CAD build for the part. Positions are in the model's coordinates, mm. Face numbers are marked on the shaded views. A direction names the side the tool comes from. Coordinates: 2 decimals unless noted, no trailing zeros. Order: outer loops, then holes, each group sorted by start corner. A loop starts at its lowest first (then second) coordinate and runs counter-clockwise, first axis right, second up. Notation, with made-up numbers: (-16.5, 84.5) - (42.5, 84.5) arc R19 ccw to (42.5, 108.5) - close; hole circle Ø6 at (24.5, 47). An arc over 180 degrees is marked (long way). Write each question's results on one line, items separated by ' | '. Start each with the question number.
Q1. Band-saw the part on B-B, the plane x = 4.5. Write the cut outline in (y, z).
Q2. Band-saw the part on A-A, the plane y = -22. Write the cut outline in (x, z).
Q3. Pin check, flat tips, straight feed: P1, Ø1.1, axis at x = 9.5, z = 59.5, coming from the -Y side; P2, Ø0.5, axis at x = 5, z = 59, coming from the +Y side; P3, Ø1, axis at y = 32.5, z = 52, coming from the -X side. Stop position of each tip, or through.
Q4. Band-saw the part on C-C, the plane z = 22.5. Write the cut outline in (x, y).
Q5. Which spindle directions (+Z, -Z, +X, -X, +Y, -Y) get a long thin tool onto all of the face, cutting with end or side? Do the marked faces 1, 2 and 3. Say none if no direction does.
Q6. Wall check: probe 1 along Z at (x, y) = (6.25, -47.5); probe 2 along X at (y, z) = (8, 29.5); probe 3 along X at (y, z) = (-48, 61.5). Give the ranges that are in metal, low to high.
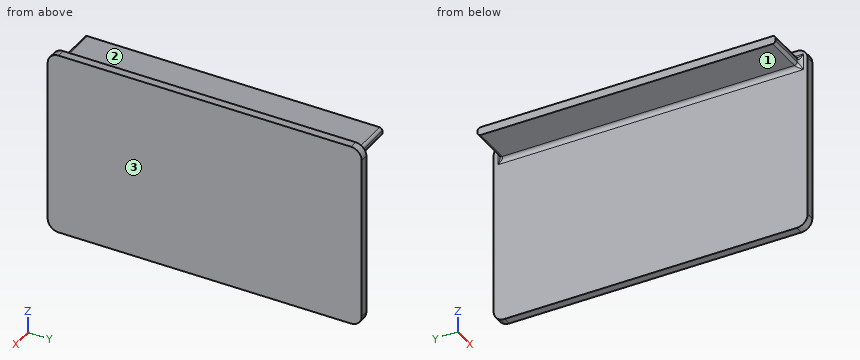
Autodesk Fusion 360 part; units mm, degrees
sketch "Boceto1" plane through (0, 0, 0) normal (1, 0, 0) x (0, 1, 0)
  line L0 (-54.5, 54) -> (54.5, 54)
  line L1 (54.5, 54) -> (54.5, 0)
  line L2 (54.5, 0) -> (-54.5, 0)
  line L3 (-54.5, 0) -> (-54.5, 54)
  dimension "d4" = 54
  dimension "d5" = 109
extrude "Extruir1" add sketch "Boceto1" along normal blind 14 makes body 1
sketch "Boceto2" plane through (0, 0, 0) normal (-1, 0, 0) x (0, -1, 0)
  line L0 (-54.5, 0) -> (54.5, 0)
  line L1 (54.5, 0) -> (54.5, 54)
  line L2 (54.5, 54) -> (-54.5, 54)
  line L3 (-54.5, 54) -> (-54.5, 0)
  line L4 (-58, -3.5) -> (-58, 64.2)
  line L5 (-58, 64.2) -> (-51.5, 64.2)
  line L6 (-51.5, 64.2) -> (-51.5, 61.2)
  line L7 (-51.5, 61.2) -> (-55, 61.2)
  line L8 (-55, 61.2) -> (-55, 57.5)
  line L9 (-55, 57.5) -> (-51.5, 57.5)
  line L10 (-51.5, 57.5) -> (-51.5, 54.5)
  line L11 (-51.5, 54.5) -> (-55, 54.5)
  line L12 (-55, 54.5) -> (-55, -0.5)
  line L13 (-55, -0.5) -> (0, -0.5)
  line L14 (-58, -3.5) -> (0, -3.5)
  line L15 (0, 2.5) -> (0, 20)
  line L16 (58, -3.5) -> (0, -3.5)
  line L17 (55, -0.5) -> (0, -0.5)
  line L18 (55, 54.5) -> (55, -0.5)
  line L19 (58, -3.5) -> (58, 64.2)
  line L20 (51.5, 54.5) -> (55, 54.5)
  line L21 (51.5, 57.5) -> (51.5, 54.5)
  line L22 (55, 57.5) -> (51.5, 57.5)
  line L23 (55, 61.2) -> (55, 57.5)
  line L24 (51.5, 61.2) -> (55, 61.2)
  line L25 (51.5, 64.2) -> (51.5, 61.2)
  line L26 (58, 64.2) -> (51.5, 64.2)
  line L27 (51.5, 64.2) -> (-51.5, 64.2)
  dimension "d10" = 0.5
  dimension "d11" = 3.7
  dimension "d12" = 3.5
  dimension "d13" = 0.5
  dimension "d14" = 0.5
  dimension "d15" = 3
  dimension "d16" = 3
  dimension "d17" = 3
  dimension "d18" = 3
extrude "Extruir2" add sketch "Boceto2" along normal blind 0 and the other way blind 16 separate body contours L4 L5 L6 L7 L8 L9 L10 L11 L12 L13 L14 L16 L17 L18 L19 L20 L21 L22 L23 L24 L25 L26 makes body 2
extrude "Extruir3" add sketch "Boceto2" along normal blind 3 contours L0 L1 L2 L3 | L4 L5 L6 L7 L8 L9 L10 L11 L12 L13 L14 L16 L17 L18 L19 L20 L21 L22 L23 L24 L25 L26 | L6 L7 L8 L9 L10 L11 L12 L13 L17 L18 L20 L21 L22 L23 L24 L25 L27 bodies 2
fillet "Empalme1" radius 4 4 edges at (6.5, 58, 64.2) (6.5, 58, -3.5) (6.5, -58, 64.2) (6.5, -58, -3.5) on bodies 2
fillet "Empalme2" radius 0.5 8 edges at (8, 51.5, 64.2) (8, 51.5, 54.5) (8, 51.5, 57.5) (8, 51.5, 61.2) (8, -51.5, 54.5) (8, -51.5, 61.2) (8, -51.5, 64.2) (8, -51.5, 57.5) on bodies 2
sketch "Boceto3" plane through (0, 0, 0) normal (0, 1, 0) x (1, 0, 0)
  line L0 (19.3, -64.2) -> (16.3, -64.2)
  line L1 (16.3, -64.2) -> (16.3, 3.5)
  line L2 (16.3, 3.5) -> (19.3, 3.5)
  line L3 (19.3, 3.5) -> (19.3, -64.2)
  line L4 (16.3, -60.85) -> (0.6, -60.85)
  line L5 (0.6, -60.85) -> (0.6, -57.85)
  line L6 (0.6, -57.85) -> (16.3, -57.85)
  line L7 (16.3, -57.85) -> (16.3, -60.85)
  line L8 (0, -61.2) -> (0, -57.5)
  line L9 (16, -61.2) -> (0, -61.2)
  point P0 (16, 3.5)
  point P1 (16, -64.2)
  dimension "d29" = 3
  dimension "d30" = 0.6
  dimension "d31" = 0.35
  dimension "d32" = 0.3
  dimension "d33" = 3
extrude "Extruir4" add sketch "Boceto3" along normal mid plane 109 separate body contours L1 L4 L5 L6 L7 makes body 3
extrude "Extruir5" add sketch "Boceto3" along normal mid plane 115 contours L0 L1 L2 L3 L7 bodies 3
fillet "Empalme3" radius 4 4 edges at (17.8, 57.5, 64.2) (17.8, -57.5, 64.2) (17.8, -57.5, -3.5) (17.8, 57.5, -3.5) on bodies 3
fillet "Empalme4" radius 1.5 4 edges at (16.3, 0, 57.85) (16.3, -54.5, 59.35) (16.3, 0, 60.85) (16.3, 54.5, 59.35) on bodies 3
fillet "Empalme5" radius 1 8 edges at (7.7, 54.5, 60.85) (15.8607, 54.9393, 61.2893) (15.8607, 54.9393, 57.4107) (7.7, 54.5, 57.85) (15.8607, -54.9393, 61.2893) (7.7, -54.5, 60.85) (7.7, -54.5, 57.85) (15.8607, -54.9393, 57.4107) on bodies 3
hidden bodies 1 2
equation "largo = 14 mm"
equation "ancho = 109 mm"
equation "alto = 54 mm"
equation "d4 = alto"
equation "d5 = ancho"
equation "d6 = largo"
equation "d21 = largo + 2 mm"
equation "d36 = ancho"
equation "d38 = ancho + 6 mm"
Results below:
1) outline: (-54.5, 58.85) arc R1 ccw to (-53.5, 57.85) - (53.5, 57.85) arc R1 ccw to (54.5, 58.85) - (54.5, 59.85) arc R1 ccw to (53.5, 60.85) - (-53.5, 60.85) arc R1 ccw to (-54.5, 59.85) - close
2) outline: (0.6, 57.85) - (14.8, 57.85) arc R1.5 cw to (16.3, 56.35) - (16.3, -3.5) - (19.3, -3.5) - (19.3, 64.2) - (16.3, 64.2) - (16.3, 62.35) arc R1.5 cw to (14.8, 60.85) - (0.6, 60.85) - close
3) P1: stops at y = -54.5 | P2: stops at y = 54.5 | P3: stops at x = 16.3
4) outline: (16.3, -57.5) - (19.3, -57.5) - (19.3, 57.5) - (16.3, 57.5) - close
5) face 1: -Z, -X, +Y, -Y | face 2: +Z, -X, +Y, -Y | face 3: +Z, -Z, +X, +Y, -Y
6) probe 1: z = 57.85 to 60.85 | probe 2: x = 16.3 to 19.3 | probe 3: x = 16.04 to 19.3
